```python
from build123d import *

# Parameters (mm, degrees)
EXTRUDE_1_DEPTH                   = 60
HOLE_WIZARD_8_5_8_5_1_D           = 8.5
HOLE_WIZARD_8_5_8_5_1_ON_FACE_2_D = 8.5


with BuildPart() as part:
    # 草图1 → 凸台-拉伸1 (new body)
    with BuildSketch(Plane.XY):
        Polygon((0, 40), (0, 0), (51, 0), (51, 10), (10, 10), (10, 40), align=None)
    extrude(amount=EXTRUDE_1_DEPTH)

    # Ø8.5 (8.5) 直径孔1 (through all)
    with Locations(Plane(origin=(10, 20, 42.5), x_dir=(0, 0, 1), z_dir=(1, 0, 0))):
        with Locations((0, 0), (-25, 0)):
            Hole(HOLE_WIZARD_8_5_8_5_1_D / 2)

    # Ø8.5 (8.5) 直径孔1 on face 2 (through all)
    with Locations(Plane(origin=(31, 10, 50), x_dir=(0, 0, 1), z_dir=(0, 1, 0))):
        with Locations((0, 0), (-40, 0)):
            Hole(HOLE_WIZARD_8_5_8_5_1_ON_FACE_2_D / 2)


solid = part.part
```
Geometry: final body of the model. Coordinates: model frame, mm. A direction names the side the tool comes from. Give positions to 0.01 mm unless a question says otherwise; leave off trailing zeros. Order: outer loops, then holes, each group sorted by start corner. A loop starts at its lowest first (then second) coordinate and runs counter-clockwise, first axis right, second up. Notation, with made-up numbers: (-31, 50.25) -> (-23, 50.25) arc R20 ccw to (-23, 56.25) -> close; hole circle Ø7 at (22.25, 68). An arc over 180 degrees is marked (long way). Write each question's results on one line, items separated by ' | '. Start each with the question number.
1) Set-up query: faces 1 (the flat face through (14, 7, 0)), 2 (the flat face through (31, 10, 30)). Return all of +Z, -Z, +X, -X, +Y, -Y with unobstructed straight access to the full face (end or side cutting, diameter ignored); none if empty.
2) Section A-A (y = 22). Return loops of the section in (x, z), then the cut area to 3 significant figures.
3) Section C-C (x = 31). Return loops of the section in (y, z).
4) Line query: line 1 (Z direction, x = 5.25, y = 20); line 2 (X direction, y = 7.5, z = 10); line 3 (Y direction, x = 3, z = 42.5). Output: solid intervals per line, ascending. Write a range as from..to.
5) Draft query along Y for faces 3 (the flat face through (5, 40, 30)), 4 (the cylindrical face through (4.93, 22.59, 45.87)), 5 (the cylindrical face through (31.187, 4.93, 54.246)). Return one class per face: pulls with the +Y half, pulls with the -Y half, needs draft (parallel to the pull), parting line crosses it, or undercut.
6) Section B-B (z = 42.5). Return loops of the section in (x, y).
7) Section D-D (y = 9). Return loops of the section in (x, z), then the cut area to 3 significant figures.
8) First-contact query: pin 1 (2 mm diameter, centred on x = 5.5, z = 13, fed in from -Y); pin 2 (1 mm diameter, centred on y = 15, z = 50.5, fed in from +X); pin 3 (13.5 mm diameter, centred on x = 31, z = 10, fed in from +Y). Flat tips, straight axial feed; report the tip coordinate or a pass-through.
Calculated:
1) face 1: -Z, +X, -X, +Y, -Y | face 2: +Z, -Z, +X, +Y
2) outline: (0, 0) -> (10, 0) -> (10, 13.75) -> (0, 13.75) -> close; (0, 21.25) -> (10, 21.25) -> (10, 38.75) -> (0, 38.75) -> close; (0, 46.25) -> (10, 46.25) -> (10, 60) -> (0, 60) -> close | area: 450 mm2
3) outline: (0, 0) -> (10, 0) -> (10, 5.75) -> (0, 5.75) -> close; (0, 14.25) -> (10, 14.25) -> (10, 45.75) -> (0, 45.75) -> close; (0, 54.25) -> (10, 54.25) -> (10, 60) -> (0, 60) -> close
4) line 1: 0..13.25, 21.75..38.25, 46.75..60 | line 2: 0..26.75, 35.25..51 | line 3: 0..15.75, 24.25..40
5) face 3: pulls with the +Y half | face 4: undercut | face 5: needs draft
6) outline: (0, 0) -> (51, 0) -> (51, 10) -> (10, 10) -> (10, 15.75) -> (0, 15.75) -> close; (0, 24.25) -> (10, 24.25) -> (10, 40) -> (0, 40) -> close
7) outline: (0, 0) -> (51, 0) -> (51, 60) -> (0, 60) -> close; hole circle Ø8.5 at (31, 10); hole circle Ø8.5 at (31, 50) | area: 2,950 mm2
8) pin 1: y = 0 | pin 2: x = 10 | pin 3: y = 10
